Check sheet for the modelled part. Datum: model origin and axes. Units: mm. Round coordinates to 2 decimals unless told otherwise and drop trailing zeros. Order: outer loops, then holes, each group sorted by start corner. A loop starts at its lowest first (then second) coordinate and runs counter-clockwise, first axis right, second up.
Q1. Depth check by flat-ended pin: P1, Ø2.5, axis at x = 11.26, z = -6.5, coming from the +Y side; P2, Ø1.5, axis at y = 1.5, z = 1.5, coming from the +X side. Enter the tip coordinate at first touch or a pass-through.
Q2. Cross-section at D-D on z = 13. Record the cut outline in (x, y).
Q3. Cross-section at B-B on z = -12. Record the cut outline in (x, y).
Q4. Cross-section at A-A on x = 0. Record the cut outline in (y, z), then the cut area to 3 significant figures.
Q5. Cross-section at C-C on z = 2.25. Record the cut outline in (x, y).
Q6. Scan lines: probe 1 along X at (y, z) = (0.7, -6.5); probe 2 along X at (y, z) = (0.85, 3); probe 3 along Z at (x, y) = (-0.5, 0.45). Record each from-to range of solid material in increasing order.
Q7. Mould release check, pull along X, two halves, no side actions. Record for faces 1 (the cylindrical face through (11.78, 1.48, 6.57)), 2 (the cylindrical face through (0, 1, -15)), 3 (the cylindrical face through (-14.054, 1.521, -8.157)): +X half, -X half, draft (parallel to the pull), parting line (faces both ways), or undercut.
from build123d import *

# Parameters (mm, degrees)
SKETCH_1_R      = 15
SKETCH_1_R_2    = 1.45
SKETCH_1_R_3    = 1.5
SKETCH_1_R_4    = 1
EXTRUDE_1_DEPTH = 3
CHAMFER_1_SIZE  = 1
SKETCH_2_R      = 3.25
SKETCH_2_R_2    = 1.45
EXTRUDE_2_DEPTH = 3
CHAMFER_2_SIZE  = 1.55
FILLET_1_R      = 2


with BuildPart() as part:
    # 草图1 → 凸台-拉伸1 (new body)
    with BuildSketch(Plane(origin=(0, 0, 0), x_dir=(1, 0, 0), z_dir=(0, 1, 0))):
        Circle(SKETCH_1_R)
        with Locations((0, -13)):
            Circle(SKETCH_1_R_2, mode=Mode.SUBTRACT)
        with Locations((-11.258330249, 6.5)):
            Circle(SKETCH_1_R_2, mode=Mode.SUBTRACT)
        with Locations((11.258330249, 6.5)):
            Circle(SKETCH_1_R_2, mode=Mode.SUBTRACT)
        with Locations((0, 12)):
            Circle(SKETCH_1_R_3, mode=Mode.SUBTRACT)
        with Locations((10.392304845, -6)):
            Circle(SKETCH_1_R_3, mode=Mode.SUBTRACT)
        with Locations((-10.392304845, -6)):
            Circle(SKETCH_1_R_3, mode=Mode.SUBTRACT)
        with Locations((0, 4.5)):
            Circle(SKETCH_1_R_4, mode=Mode.SUBTRACT)
        with Locations((3.897114317, -2.25)):
            Circle(SKETCH_1_R_4, mode=Mode.SUBTRACT)
        with Locations((-3.897114317, -2.25)):
            Circle(SKETCH_1_R_4, mode=Mode.SUBTRACT)
        Circle(SKETCH_1_R_3, mode=Mode.SUBTRACT)
    extrude(amount=EXTRUDE_1_DEPTH)

    # 倒角1
    chamfer_1_edges = [part.edges().sort_by_distance(p)[0] for p in [
        (-1, 0, -4.5),
        (2.897114317, 0, 2.25),
        (-4.897114317, 0, 2.25),
    ]]
    chamfer(chamfer_1_edges, length=CHAMFER_1_SIZE)

    # 草图2 → 凸台-拉伸2 (add)
    with BuildSketch(Plane(origin=(0, 3, 0), x_dir=(1, 0, 0), z_dir=(0, 1, 0))):
        with Locations((11.258330249, 6.5)):
            Circle(SKETCH_2_R)
        with Locations((11.258330249, 6.5)):
            Circle(SKETCH_2_R_2, mode=Mode.SUBTRACT)
        with Locations((0, -13)):
            Circle(SKETCH_2_R)
        with Locations((0, -13)):
            Circle(SKETCH_2_R_2, mode=Mode.SUBTRACT)
        with Locations((-11.258330249, 6.5)):
            Circle(SKETCH_2_R)
        with Locations((-11.258330249, 6.5)):
            Circle(SKETCH_2_R_2, mode=Mode.SUBTRACT)
    extrude(amount=-EXTRUDE_2_DEPTH)

    # 倒角2
    chamfer_2_edges = [part.edges().sort_by_distance(p)[0] for p in [
        (9.808330249, 3, -6.5),
        (-1.45, 3, 13),
        (-12.708330249, 3, -6.5),
    ]]
    chamfer(chamfer_2_edges, length=CHAMFER_2_SIZE)

    # 圆角1
    fillet_1_edges = [part.edges().sort_by_distance(p)[0] for p in [
        (11.401719222, 1.5, -9.746835321),
        (14.141866606, 1.5, -5.000760833),
        (2.740147383, 1.5, 14.747596154),
        (-2.740147383, 1.5, 14.747596154),
        (-11.401719222, 1.5, -9.746835321),
        (-14.141866606, 1.5, -5.000760833),
    ]]
    fillet(fillet_1_edges, radius=FILLET_1_R)


solid = part.part
Results found:
1. P1: passes through
1. P2: stops at x = 14.98
2. outline: (-7.48, 0) - (-1.45, 0) - (-1.45, 1.45) - (-3, 3) - (-7.48, 3) - close; (1.45, 0) - (7.48, 0) - (7.48, 3) - (3, 3) - (1.45, 1.45) - close
3. outline: (-9, 0) - (-1.5, 0) - (-1.5, 3) - (-9, 3) - close; (1.5, 0) - (9, 0) - (9, 3) - (1.5, 3) - close
4. outline: (0, -15) - (3, -15) - (3, -13.5) - (0, -13.5) - close; (0, -10.5) - (3, -10.5) - (3, -5.5) - (1, -5.5) - (0, -6.5) - close; (0, -2.5) - (1, -3.5) - (3, -3.5) - (3, -1.5) - (0, -1.5) - close; (0, 1.5) - (3, 1.5) - (3, 10) - (1.45, 11.55) - (0, 11.55) - close; (0, 14.45) - (1.45, 14.45) - (3, 16) - (3, 16.25) - (0, 16.25) - close
4. area: 57.6 mm2
5. outline: (-14.83, 0) - (-5.9, 0) - (-4.9, 1) - (-4.9, 3) - (-14.83, 3) - close; (-2.9, 1) - (-1.9, 0) - (1.9, 0) - (2.9, 1) - (2.9, 3) - (-2.9, 3) - close; (4.9, 1) - (5.9, 0) - (14.83, 0) - (14.83, 3) - (4.9, 3) - close
6. probe 1: x = -14.51 to -12.71, -9.81 to 9.81, 12.71 to 14.51
6. probe 2: x = -14.7 to -4.77, -3.03 to 3.03, 4.77 to 14.7
6. probe 3: z = -14.99 to -13.41, -10.59 to -5.97, -3.03 to -1.41, 1.41 to 11.64, 14.36 to 16.21
7. face 1: undercut
7. face 2: parting line
7. face 3: -X half
